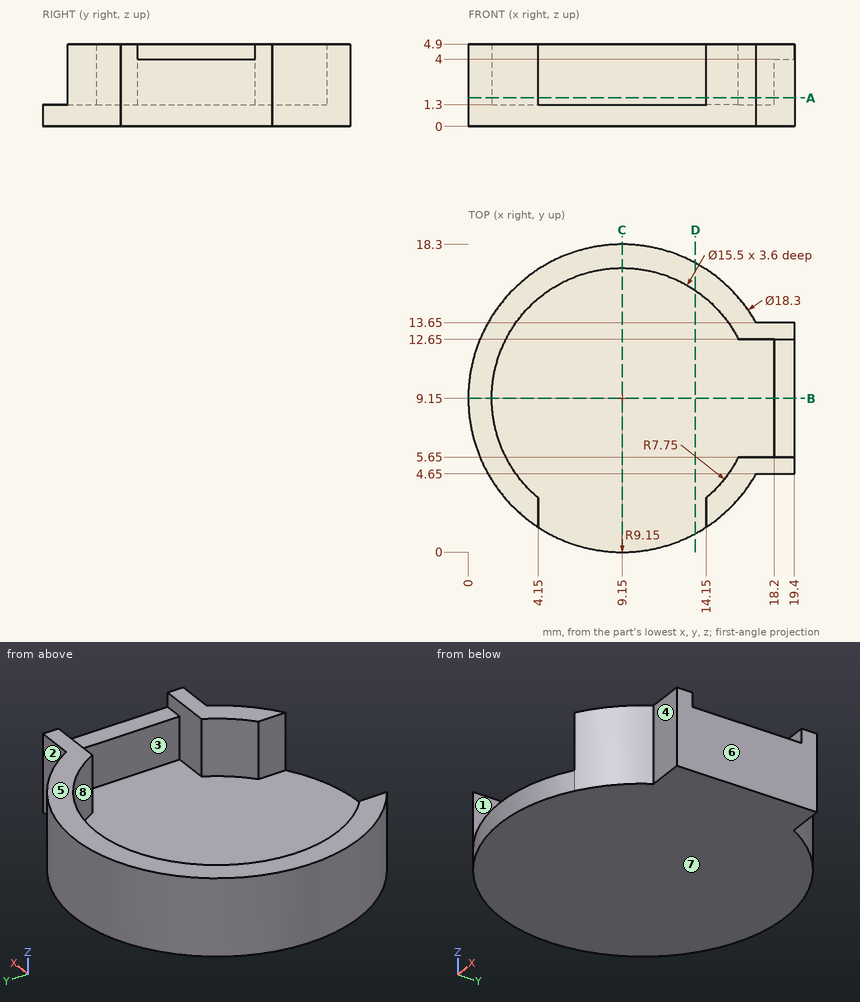
Could you check a few things on this drawing? It's one solid part, dimensions in mm from its lowest x, y, z. A direction names the side the tool comes from. Coordinates: 2 decimals unless noted, no trailing zeros. Write each loop counter-clockwise with the first axis right and the second up, starting at its lowest first coordinate (ties: lowest second). Pieces come first, ordered by that corner, then holes.
1) If we section it at D-D (x = 13.5): List the corners of the cut face in (y, z) for me.
Filled in:
outline: (1.1, 0) - (17.2, 0) - (17.2, 4.9) - (15.56, 4.9) - (15.56, 1.3) - (1.1, 1.3) - close
2) If I drill on line 1 (X direction, y = 9.15, z = 2.45); line 2 (Y direction, x = 17.25, z = 2.55); line 3 (X direction, y = 13, z = 3.2), over which ranges is the centre line in solid material (lowest first)?
Filled in:
line 1: x = 0 to 1.4, 18.2 to 19.4
line 2: y = 4.65 to 5.65, 12.65 to 13.65
line 3: x = 0.85 to 2.42, 15.88 to 19.4
3) Thinking about a two-plate mould opening in X: for the marked faces 6, 7 and 8, which applies, +X half, -X half, draft (parallel to the pull), parting line (faces both ways), or undercut?
Filled in:
face 6: +X half
face 7: draft
face 8: undercut
4) I'm going to push flat-ended pins straight in: pin 1 (1 mm diameter, centred on x = 17, z = 2.5, fed in from +Y); pin 2 (0.9 mm diameter, centred on y = 2, z = 3, fed in from -X); pin 3 (1.1 mm diameter, centred on x = 18.5, z = 1.5, fed in from +Y). Where does each tip first touch, or does it pass through?
Filled in:
pin 1: stops at y = 14.6
pin 2: stops at x = 2.92
pin 3: stops at y = 13.65
5) Which directions (+Z, -Z, +X, -X, +Y, -Y) give clear straight access to the entire face, cutting with the end or side of a thin tool? Please do the marked faces 1, 2, 3, 4 and 5.
Filled in:
face 1: +Z, -Y
face 2: +Z, -Z, +X, +Y
face 3: +Z
face 4: +Z, -Z, +X, -Y
face 5: +Z, +X, -X, +Y, -Y
6) If we section it at B-B (y = 9.15): List the corners of the cut face in (x, z) for me, plus the area to 3 significant figures.
Filled in:
outline: (0, 0) - (19.4, 0) - (19.4, 4) - (18.2, 4) - (18.2, 1.3) - (1.4, 1.3) - (1.4, 4.9) - (0, 4.9) - close
area: 33.5 mm2
7) If we section it at A-A (z = 1.7): List the corners of the cut face in (x, y) for me.
Filled in:
outline: (4.15, 1.49) - (4.15, 3.23) arc R7.75 cw (long way) to (16.06, 12.65) - (18.2, 12.65) - (18.2, 5.65) - (16.06, 5.65) arc R7.75 cw to (14.15, 3.23) - (14.15, 1.49) arc R9.15 ccw to (17.12, 4.65) - (19.4, 4.65) - (19.4, 13.65) - (17.12, 13.65) arc R9.15 ccw (long way) to start
8) If we section it at C-C (x = 9.15): List the corners of the cut face in (y, z) for me.
Filled in:
outline: (0, 0) - (18.3, 0) - (18.3, 4.9) - (16.9, 4.9) - (16.9, 1.3) - (0, 1.3) - close
